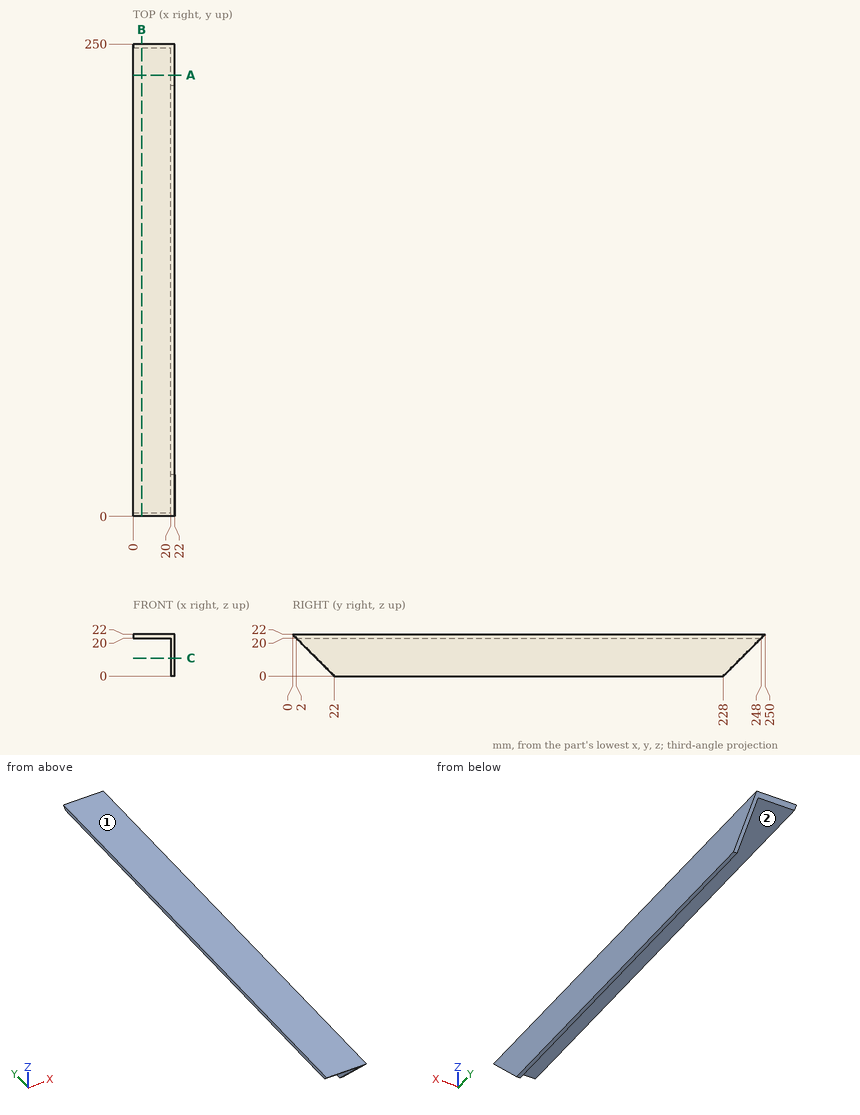
Verification items for this drawing (mm, ordinates from the low corner). A direction names the side the tool comes from. Coordinates: 2 decimals unless noted, no trailing zeros. Order: outer loops, then holes, each group sorted by start corner. A loop starts at its lowest first (then second) coordinate and runs counter-clockwise, first axis right, second up. Notation, with made-up numbers: M 21.5,83.5 L 44.5,83.5 A32 cw 44.5,113.5 Z; hole C 39.5,-15.5 d8. An arc over 180 degrees is marked long. One line per item, written item: value. Start each with the question number.
Item 1: Sectioned sample at B-B on x = 4.5. Record the cut outline in (y, z), then the cut area to 3 significant figures.
Item 2: Access from +Z, -Z, +X, -X, +Y, -Y to the whole of each face (thin tool, end or side, straight path). Record for the marked faces 1 and 2.
Item 3: Depth check by flat-ended pin: P1, Ø6, axis at x = 8.5, y = 165, coming from the -Z side; P2, Ø8, axis at y = 58.5, z = 4, coming from the -X side. Enter the tip coordinate at first touch or a pass-through.
Item 4: Sectioned sample at C-C on z = 9.5. Record the cut outline in (x, y), then the cut area to 3 significant figures.
Item 5: Thickness scan on probe 1 along Z at (x, y) = (9, 82.5); probe 2 along Y at (x, z) = (20.25, 14.5). Record the ranges inside material, lowest first.
Item 6: Sectioned sample at A-A on y = 233.5. Record the cut outline in (x, z), then the cut area to 3 significant figures.
Calculated:
1. outline: M 0,22 L 2,20 L 248,20 L 250,22 Z
1. area: 496 mm^2
2. face 1: +Z, +X, -X, +Y, -Y
2. face 2: -Z, -X, +Y, -Y
3. P1: z = 20
3. P2: x = 20
4. outline: M 20,12.5 L 22,12.5 L 22,237.5 L 20,237.5 Z
4. area: 450 mm^2
5. probe 1: 20 to 22
5. probe 2: 7.5 to 242.5
6. outline: M 0,20 L 20,20 L 20,5.5 L 22,5.5 L 22,22 L 0,22 Z
6. area: 73.0 mm^2
